from build123d import *

# Parameters (mm, degrees)
F1_DEPTH = 173
F3_DEPTH = 43
F5_DEPTH = 43
F6_W     = 1.6
F6_H     = 75
F7_DEPTH = 30
F8_R     = 4
F9_DEPTH = 432.001
F10_R    = 5


with BuildPart() as f1:
    # F0 (on Right) → F1 (new body, symmetric)
    with BuildSketch(Plane.YZ):
        Polygon((0, 94), (0, 0), (0, -94), (50, -94), (50, -64), (48.4, -64), (48.4, -92.4), (1.6, -92.4), (1.6, 92.4), (48.4, 92.4), (48.4, 64), (50, 64), (50, 94), align=None)
    extrude(amount=F1_DEPTH, both=True)

    # F2 (on face) → F3 (join)
    with BuildSketch(Plane.YZ.offset(173)):
        Polygon((0, 37.5), (0, 0), (0, -37.5), (1.6, -37.5), (1.6, 37.5), align=None)
    extrude(amount=F3_DEPTH)

    # F4 (on face) → F5 (join)
    with BuildSketch(Plane(origin=(-173, 0, 0), x_dir=(0, -1, 0), z_dir=(-1, 0, 0))):
        Polygon((0, -37.5), (0, 0), (0, 37.5), (-1.6, 37.5), (-1.6, -37.5), align=None)
    extrude(amount=F5_DEPTH)

    # F6 (on face) → F7 (join)
    with BuildSketch(Plane(origin=(0, 1.6, 0), x_dir=(-1, 0, 0), z_dir=(0, 1, 0))):
        with Locations((-215.2, 0)):
            Rectangle(F6_W, F6_H)
        with Locations((215.2, 0)):
            Rectangle(F6_W, F6_H)
    extrude(amount=F7_DEPTH)

    # F8 (on face) → F9 (cut, through all)
    with BuildSketch(Plane.YZ.offset(216)):
        with Locations((16.6, 22.5)):
            Circle(F8_R)
        with Locations((16.6, -22.5)):
            Circle(F8_R)
    extrude(amount=-F9_DEPTH, mode=Mode.SUBTRACT)

    # F10
    f10_edges = [f1.edges().sort_by_distance(p)[0] for p in [
        (173, 0.8, 37.5),
        (215.2, 31.6, -37.5),
        (173, 0.8, -37.5),
        (173, 49.2, 64),
        (173, 49.2, -64),
        (215.2, 31.6, 37.5),
        (-173, 49.2, -64),
        (-173, 0.8, -37.5),
        (-215.2, 31.6, -37.5),
        (-215.2, 31.6, 37.5),
        (-173, 0.8, 37.5),
        (-173, 49.2, 64),
        (0, 50, -94),
        (0, 0, -94),
        (-216, 0, 0),
        (0, 1.6, -92.4),
        (0, 48.4, -92.4),
        (-214.4, 1.6, 0),
        (214.4, 1.6, 0),
        (216, 0, 0),
        (0, 0, 94),
        (0, 50, 94),
        (0, 48.4, 92.4),
        (0, 1.6, 92.4),
    ]]
    fillet(f10_edges, radius=F10_R)


solid = f1.part
Source: CAD feature listing. Evaluate the final solid. Frame: model axes, mm. A direction names the side the tool comes from. Coordinates: 2 decimals unless noted, no trailing zeros. Write each loop counter-clockwise with the first axis right and the second up, starting at its lowest first coordinate (ties: lowest second). Pieces come first, ordered by that corner, then holes. Notation, with made-up numbers: M -0.75,-4.5 L 9.25,-4.5 A21 cw 9.25,0.5 Z; hole C 27.5,-21 d5. An arc over 180 degrees is marked long. Use a Markdown table: item, result.
1) Section D-D, the plane z = -52. Output: boundary loops of the cut face in (x, y), then the cut area to 3 significant figures.
Conclusion:
| item | result |
|---|---|
| outline | M -173,0 L 173,0 L 173,1.6 L -173,1.6 Z |
| area | 554 mm^2 |
2) Section C-C, the plane x = 48.5. Output: boundary loops of the cut face in (y, z), then the cut area to 3 significant figures.
Conclusion:
| item | result |
|---|---|
| outline | M 0,-89 A5 ccw 5,-94 L 45,-94 A5 ccw 50,-89 L 50,-64 L 48.4,-64 L 48.4,-87.4 A5 cw 43.4,-92.4 L 6.6,-92.4 A5 cw 1.6,-87.4 L 1.6,87.4 A5 cw 6.6,92.4 L 43.4,92.4 A5 cw 48.4,87.4 L 48.4,64 L 50,64 L 50,89 A5 ccw 45,94 L 5,94 A5 ccw 0,89 Z |
| area | 547 mm^2 |
3) First-contact query: pin 1 Ø5 at (y, z) = (16.6, -22.5) entering from -X; pin 2 Ø1.3 at (x, y) = (42.5, 49.5) entering from +Z; pin 3 Ø25 at (y, z) = (15, -81) entering from +X; pin 4 Ø1.8 at (x, z) = (-215.5, -12) entering from +Y. Flat tips, straight axial feed; report the tip coordinate or a pass-through.
Conclusion:
| item | result |
|---|---|
| pin 1 | passes through |
| pin 2 | stops at z = 92.19 |
| pin 3 | stops at x = 173 |
| pin 4 | stops at y = 31.6 |
4) Section A-A, the plane y = 16.6. Give the number of separate pieces and of enclosed holes in the cut face, then the cut area to 3 significant figures.
Conclusion:
| item | result |
|---|---|
| separate pieces | 8 |
| enclosed holes | 0 |
| area | 1,300 mm^2 |
5) Section B-B, the plane z = 79. Output: boundary loops of the cut face in (x, y), then the cut area to 3 significant figures.
Conclusion:
| item | result |
|---|---|
| outline | M -173,0 L 173,0 L 173,1.6 L -173,1.6 Z; M -173,48.4 L 173,48.4 L 173,50 L -173,50 Z |
| area | 1,110 mm^2 |
6) Reachability of faces 1 (the flat face through (2, 25, 92.4)), 2 (the flat face through (-203, 1, -37.5)), 3 (the flat face through (-203, 1, 37.5)) from +Z, -Z, +X, -X, +Y, -Y: full face, straight path, thin tool, end or side. Return the list, or none.
Conclusion:
| item | result |
|---|---|
| face 1 | +X, -X |
| face 2 | -Z, -X, +Y, -Y |
| face 3 | +Z, -X, +Y, -Y |
7) Ray query, L1, parallel to Z at x = -214.8, y = 16.6; L2, parallel to Z at x = 153.5, y = 25; L3, parallel to X at y = 28.5, z = 21. Return the intervals inside material, ascending.
Conclusion:
| item | result |
|---|---|
| L1 | z = -37.5 to -26.5, -18.5 to 18.5, 26.5 to 37.5 |
| L2 | z = -94 to -92.4, 92.4 to 94 |
| L3 | x = -216 to -214.4, 214.4 to 216 |
8) Mould query, pull axis Y, two halves, no side actions, for faces 4 (the flat face through (2, 25, -92.4)), 5 (the cylindrical face through (215.211, 18.75, 25.873)), 6 (the flat face through (3, 0, 1)), 7 (the flat face through (173, 19, -93)). Classes: pulls with the +Y half, pulls with the -Y half, needs draft (parallel to the pull), parting line crosses it, or undercut.
Conclusion:
| item | result |
|---|---|
| face 4 | undercut |
| face 5 | undercut |
| face 6 | pulls with the -Y half |
| face 7 | needs draft |
